Autodesk Inventor part; units mm, degrees
ref_plane "Work Plane1" through (64.1405, 0, 0) normal (0, 1, 0) x (-1, 0, 0)
ref_plane "YZ Plane" through (0, 0, 0) normal (1, 0, 0) x (0, 1, 0)
ref_plane "XZ Plane" through (0, 0, 0) normal (0, 1, 0) x (-1, 0, 0)
sketch "草图1" plane through (0, 0, 0) normal (0, 0, 1) x (1, 0, 0)
  line L0 (0, 0) -> (8, 0)
  line L1 (0, 0) -> (0, 22.5)
  line L2 (0, 22.5) -> (8, 22.5)
  line L3 (8, 22.5) -> (8, 0)
  line L4 (0, 27) -> (0, -4.5)
  line L5 (-1.6, 0) -> (9.6, 0)
  dimension "d1" = 45
  dimension "d2" = 8
revolve "轴承体" add sketch "草图1" angle 360 about axis through (0, 0, 0) along (1, 0, 0)
sketch "草图2" plane through (0, 0, 0) normal (-1, 0, 0) x (0, 0, 1)
  circle A0 centre (0, 0) radius 22.5
  point P0 (0, 0)
hole "螺纹" at (0, 0, 0) direction (1, 0, 0) diameter 28.376 end through all
sketch "草图3" plane through (8, 0, 0) normal (1, 0, 0) x (0, 0, -1)
  circle A0 centre (0, 0) radius 22.5
  line L0 (-2.5, 22.3607) -> (-2.5, 20)
  line L1 (-2.5, 20) -> (2.5, 20)
  line L2 (2.5, 20) -> (2.5, 22.3607)
  line L3 (0, -31.5) -> (0, 31.5)
  line L4 (-31.5, 0) -> (31.5, 0)
  dimension "d12" = 2.5
  dimension "d13" = 2.5
  dimension "d14" = 20
extrude "沟槽1" cut sketch "草图3" against normal through all contours L2 L1 L3 A0 | L3 L1 L0 A0
pattern_circular "IDS_ARRAYGROOVE{1}" count 4 over 360 about axis through (-10, 0, 0) along (1, 0, 0) of "沟槽1"
chamfer "倒角1" distance 1 angle 45 4 edges at (0, 15.9099, -15.9099) (0, 15.9099, 15.9099) (0, -15.9099, -15.9099) (0, -15.9099, 15.9099) measured on face at (0, -17.8541, -8.1385)
chamfer "倒角2" distance 1 angle 45 4 edges at (8, 15.9099, 15.9099) (8, 15.9099, -15.9099) (8, -15.9099, -15.9099) (8, -15.9099, 15.9099) measured on face at (8, -17.8541, -8.1385)
chamfer "倒角3" distance 0.75 angle 30 1 edges at (8, 0, -14.188) measured on face at (8, 17.2423, 7.8853)
chamfer "倒角4" distance 0.75 angle 30 1 edges at (0, 0, -14.188) measured on face at (0, 17.2423, 7.8853)
ref_plane "Work Plane1" through (64.1405, 0, 0) normal (0, 1, 0) x (-1, 0, 0)
equation "\"d1\" = SD2"
equation "\"d2\" = KOH"
equation "\"d12\" = 0.5 * SNB"
equation "\"d13\" = 0.5 * SNB"
equation "\"d14\" = 0.5 * SD2 - SNT"
equation "\"d10\" = -0.5 * LADI + 0.5 * SD2"
equation "\"d11\" = FAWI"
equation "\"d41\" = -0.5 * LADI + 0.5 * SD2"
equation "\"d25\" = -0.5 * LADI + 0.5 * SD2"
equation "\"d27\" = FAWI"
equation "\"d42\" = -0.5 * LADI + 0.5 * SD2"
equation "\"d18\" = 0.025 * NND"
equation "\"d43\" = 0.025 * NND"
equation "\"d20\" = 0.025 * NND"
equation "\"d44\" = 0.025 * NND"
equation "\"KOH\" = 8"
equation "\"SD2\" = 45"
equation "\"SNB\" = 5"
equation "\"SNT\" = 2.5"
equation "\"LADI\" = 43"
equation "\"FAWI\" = 45deg"
equation "\"GUL\" = 0.61345 * PTC"
equation "\"PHH\" = 1"
equation "\"TOA\" = 30deg"
equation "\"PTC\" = 1.5"
equation "\"FAWI1\" = 60deg"
equation "\"GAL\" = 0.61345 * PTC"
equation "\"GD1\" = THREADDIA - 1.2269 * PTC"
properties part number "螺母 GB 810 M30 x 1.5" material "钢，软"
Here's how the part is built. I have some questions about the finished solid (model axes, mm). A direction names the side the tool comes from. Round coordinates to 2 decimals unless told otherwise and drop trailing zeros. Loops run counter-clockwise (first coordinate to the right, second up) from the corner with the lowest first, then second, coordinate; pieces in that order, holes last. Notation, with made-up numbers: (-22, -39) -> (4, -39) arc R8 cw to (4, -34) -> close; hole circle Ø10 at (20, 76.25). An arc over 180 degrees is marked (long way). Write each question's results on one line, items separated by ' | '.
(1) For P1, Ø0.7, axis at x = 2.5, y = 21, coming from the +Z side; P2, Ø1.9, axis at x = 2, y = 21, coming from the -Z side; P3, Ø1.9, axis at x = 5, z = 21, coming from the +Y side, each with a flat end and sliding along its axis, tell me the tip position at first contact or that it passes through.
Worked answers:
P1: z = 8.93 | P2: z = -10.21 | P3: y = 10.21
(2) We'd pull the mould along Z, two halves only. Please class faces 1 (the face through (4, 2.5, -21)), 2 (the face through (4, 0, 20)), 3 (the face through (4.04, 15.76, -16.06)), 4 (the face through (4, 20, 0)): released by +Z, released by -Z, zero draft, split by the parting line, or undercut.
Worked answers:
face 1: zero draft | face 2: released by +Z | face 3: released by -Z | face 4: undercut
(3) If we section it at A-A, the plane y = 0: List the corners of the cut face in (x, z) for me.
Worked answers:
outline: (0, -20) -> (8, -20) -> (8, -14.94) -> (7.57, -14.19) -> (0.43, -14.19) -> (0, -14.94) -> close; (0, 14.94) -> (0.43, 14.19) -> (7.57, 14.19) -> (8, 14.94) -> (8, 20) -> (0, 20) -> close
(4) If I drill on L1, parallel to Z at x = 5.25, y = 0; L2, parallel to Y at x = 5.75, z = -1.5, over which ranges is the centre line in solid material (lowest first)?
Worked answers:
L1: -20 to -14.19, 14.19 to 20 | L2: -20 to -14.11, 14.11 to 20
(5) If we section it at B-B, the plane x = 3.75: List the corners of the cut face in (y, z) for me.
Worked answers:
outline: (-22.36, -2.5) arc R22.5 ccw to (-2.5, -22.36) -> (-2.5, -20) -> (2.5, -20) -> (2.5, -22.36) arc R22.5 ccw to (22.36, -2.5) -> (20, -2.5) -> (20, 2.5) -> (22.36, 2.5) arc R22.5 ccw to (2.5, 22.36) -> (2.5, 20) -> (-2.5, 20) -> (-2.5, 22.36) arc R22.5 ccw to (-22.36, 2.5) -> (-20, 2.5) -> (-20, -2.5) -> close; hole circle Ø28.38 at (0, 0)
(6) For faces 5 (the face through (4, -21, -2.5)), 6 (the face through (4, -2.5, -21)), 7 (the face through (4, 21, 2.5)), which set-ups out of +Z, -Z, +X, -X, +Y, -Y let a thin tool reach every point of the face, with its end or its side?
Worked answers:
face 5: +X, -X, -Y | face 6: -Z, +X, -X | face 7: +X, -X, +Y
